Read the model definition and answer for the solid it produces. Units are mm, in the model's axes. A direction names the side the tool comes from. Give positions to 0.01 mm unless a question says otherwise; leave off trailing zeros. Order: outer loops, then holes, each group sorted by start corner. A loop starts at its lowest first (then second) coordinate and runs counter-clockwise, first axis right, second up. Notation, with made-up numbers: (64, 16.5) - (69, 16.5) arc R25 cw to (69, 47.5) - close; hole circle Ø4 at (5.25, 84.25). An arc over 180 degrees is marked (long way). Write item = value, one per line.
```python
from build123d import *

# Parameters (mm, degrees)
SKETCH1_R             = 13.5
BOSS_EXTRUDE1_DEPTH   = 14
BOSS_EXTRUDE2_START   = -7
SKETCH2_R             = 13.5
SKETCH2_R_2           = 12.5
BOSS_EXTRUDE2_DEPTH   = 7
F_4_0MM_DOWEL_HOLE1_D = 4
SKETCH16_W            = 100
SKETCH16_H            = 50
BOSS_EXTRUDE3_DEPTH   = 8
BOSS_EXTRUDE4_DEPTH   = 8
CHAMFER2_SIZE         = 5
SKETCH18_W            = 38
SKETCH18_H            = 65
BOSS_EXTRUDE5_DEPTH   = 44
SKETCH15_R            = 5
CUT_EXTRUDE1_DEPTH    = 86.586213843
CHAMFER3_SIZE         = 5


with BuildPart() as part:
    # Sketch1 → Boss-Extrude1 (new body)
    with BuildSketch(Plane.XY):
        Polygon((-40, 0), (-40, -35), (60, -35), (60, 3.080013472), (60, 30), (-40, 30), align=None)
        Circle(SKETCH1_R, mode=Mode.SUBTRACT)
    extrude(amount=BOSS_EXTRUDE1_DEPTH)

    # Sketch2 → Boss-Extrude2 (add)
    with BuildSketch(Plane.XY.offset(14).offset(BOSS_EXTRUDE2_START)):
        Circle(SKETCH2_R)
        Circle(SKETCH2_R_2, mode=Mode.SUBTRACT)
    extrude(amount=BOSS_EXTRUDE2_DEPTH)

    # Ø4.0mm Dowel Hole1 (through all)
    with Locations(Plane.XY.offset(14)):
        with Locations((-12, 12), (12, 12), (12, -12), (-12, -12)):
            Hole(F_4_0MM_DOWEL_HOLE1_D / 2)

    # Sketch16 → Boss-Extrude3 (add)
    with BuildSketch(Plane.XZ.offset(35)):
        with Locations((10, 25)):
            Rectangle(SKETCH16_W, SKETCH16_H)
    extrude(amount=-BOSS_EXTRUDE3_DEPTH)

    # Sketch17 → Boss-Extrude4 (add)
    with BuildSketch(Plane(origin=(60, 0, 0), x_dir=(0, 0, -1), z_dir=(1, 0, 0))):
        Polygon((-44, -27), (-14, 3), (-14, -27), align=None)
    boss_extrude4 = extrude(amount=-BOSS_EXTRUDE4_DEPTH)

    # Mirror1: Boss-Extrude4 across plane
    add(boss_extrude4.mirror(Plane(origin=(10, 0, 0), x_dir=(0, 0, 1), z_dir=(1, 0, 0))))

    # Chamfer2
    chamfer2_edges = [part.edges().sort_by_distance(p)[0] for p in [
        (-40, 30, 7),
    ]]
    chamfer(chamfer2_edges, length=CHAMFER2_SIZE)

    # Sketch18 → Boss-Extrude5 (add)
    with BuildSketch(Plane.XY.offset(50)):
        with Locations((41, -2.5)):
            Rectangle(SKETCH18_W, SKETCH18_H)
    extrude(amount=-BOSS_EXTRUDE5_DEPTH)

    # Sketch15 → Cut-Extrude1 (cut, through all)
    with BuildSketch(Plane(origin=(0, 0, 0), x_dir=(-1, 0, 0), z_dir=(0, 0, -1))):
        with Locations((-38, 5)):
            Circle(SKETCH15_R)
    extrude(amount=-CUT_EXTRUDE1_DEPTH, mode=Mode.SUBTRACT)

    # Chamfer3
    chamfer3_edges = [part.edges().sort_by_distance(p)[0] for p in [
        (60, 30, 25),
    ]]
    chamfer(chamfer3_edges, length=CHAMFER3_SIZE)


solid = part.part
```
1. For faces 1 (the face through (9, -9, 7)), 2 (the face through (-36, -12, 29)), 3 (the face through (-9, -27, 32)), determine the directions among +Z, -Z, +X, -X, +Y, -Y from which every point of the face is accessible in a straight line to the end or side of a thin tool.
Recorded:
face_1 = -Z
face_2 = +Z, -X, +Y
face_3 = +Z, +Y
2. Flat-ended cylindrical pins translate along their axes: pin 1 (3 mm diameter, centred on x = -12, y = 12, fed in from -Z); pin 2 (1 mm diameter, centred on x = -29.5, z = 31, fed in from +Y); pin 3 (8 mm diameter, centred on x = 11.5, y = 0, fed in from +Z). Find the tip coordinate at first contact, or state that the pin passes through.
Recorded:
pin_1 = through
pin_2 = -27
pin_3 = 14
3. Determine the mould class of faces 4 (the face through (-32, -18, 22)), 5 (the face through (12, 14, 7)), 6 (the face through (20.6, 30, 13.5)) for opening direction Y: +Y half, -Y half, draft (parallel to the pull), parting line (faces both ways), or undercut.
Recorded:
face_4 = draft
face_5 = undercut
face_6 = +Y half
4. Section B-B (x = 0) is taken. Determine the outline of the cut face in (y, z), and give its area (3 significant figures).
Recorded:
outline = (-35, 0) - (-13.5, 0) - (-13.5, 7) - (-12.5, 7) - (-12.5, 14) - (-27, 14) - (-27, 50) - (-35, 50) - close; (12.5, 7) - (13.5, 7) - (13.5, 0) - (30, 0) - (30, 14) - (12.5, 14) - close
area = 834 mm^2
5. Section D-D (y = 23.5) is taken. Determine the outline of the cut face in (x, z), and give its area (3 significant figures).
Recorded:
outline = (-40, 0) - (60, 0) - (60, 50) - (22, 50) - (22, 14) - (-40, 14) - close
area = 2,770 mm^2
6. Straight lines are drawn through the part: L1, parallel to Y at x = 0, z = 4.75; L2, parallel to Y at x = 0, z = 9.5; L3, parallel to X at y = 8, z = 11.5. For each, find the intervals that lie inside material, in ascending order. Write a range as [from, to].
Recorded:
L1 = [-35, -13.5], [13.5, 30]
L2 = [-35, -12.5], [12.5, 30]
L3 = [-40, -9.6], [9.6, 34], [42, 60]
7. Section C-C (z = 9.5) is taken. Determine the outline of the cut face in (x, y).
Recorded:
outline = (-40, -35) - (60, -35) - (60, 25) - (55, 30) - (-35, 30) - (-40, 25) - close; hole circle Ø4 at (-12, -12); hole circle Ø4 at (-12, 12); hole circle Ø25 at (0, 0); hole circle Ø4 at (12, -12); hole circle Ø4 at (12, 12); hole circle Ø10 at (38, 5)
8. Section A-A (z = 36.5) is taken. Determine the outline of the cut face in (x, y), and give its area (3 significant figures).
Recorded:
outline = (-40, -35) - (60, -35) - (60, 25) - (55, 30) - (22, 30) - (22, -27) - (-32, -27) - (-32, -19.5) - (-40, -19.5) - close; hole circle Ø10 at (38, 5)
area = 2,930 mm^2
